```python
from build123d import *

# Parameters (mm, degrees)
SKETCH1_W                = 12.5984
SKETCH1_H                = 13.4112
BOSS_EXTRUDE1_DEPTH      = 46.99
BOSS_EXTRUDE1_DEPTH_BACK = 39.37
SKETCH2_R                = 3.1242
CUT_EXTRUDE1_DEPTH       = 87.36
SKETCH4_R                = 2.54
BOSS_EXTRUDE2_DEPTH      = 2.54
FILLET2_R                = 0.508
FILLET2_OF_MIRROR1_R     = 0.508
FILLET1_R                = 1.778
CHAMFER1_SIZE            = 1.27


with BuildPart() as part:
    # Sketch1 → Boss-Extrude1 (new body, two sides)
    with BuildSketch(Plane(origin=(0, 0, 0), x_dir=(1, 0, 0), z_dir=(0, 1, 0))) as boss_extrude1_sk:
        with Locations((-1.1938, -0.7874)):
            Rectangle(SKETCH1_W, SKETCH1_H)
    extrude(amount=BOSS_EXTRUDE1_DEPTH)
    extrude(boss_extrude1_sk.sketch, amount=-BOSS_EXTRUDE1_DEPTH_BACK)

    # Sketch2 → Cut-Extrude1 (cut, through all)
    with BuildSketch(Plane(origin=(0, 46.99, 0), x_dir=(1, 0, 0), z_dir=(0, 1, 0))):
        with Locations(Location((0, 0, 0), (0, 0, 270))):  # turned: the seam where the file's is
            Circle(SKETCH2_R)
    extrude(amount=-CUT_EXTRUDE1_DEPTH, mode=Mode.SUBTRACT)

    # Sketch4 → Boss-Extrude2 (add)
    with BuildSketch(Plane(origin=(5.1054, 0, 0), x_dir=(0, 0, -1), z_dir=(1, 0, 0))):
        with Locations((0, -20.32)):
            Circle(SKETCH4_R)
    boss_extrude2 = extrude(amount=BOSS_EXTRUDE2_DEPTH)

    # Fillet2
    fillet2_edges = [part.edges().sort_by_distance(p)[0] for p in [
        (7.6454, -20.32, 2.54),
    ]]
    fillet(fillet2_edges, radius=FILLET2_R)

    # Mirror1: Boss-Extrude2 across plane
    add(boss_extrude2.mirror(Plane.ZX))

    # Fillet2 of Mirror1
    fillet2_of_mirror1_edges = [part.edges().sort_by_distance(p)[0] for p in [
        (7.6454, 20.32, 2.54),
    ]]
    fillet(fillet2_of_mirror1_edges, radius=FILLET2_OF_MIRROR1_R)

    # Fillet1
    fillet1_edges = [part.edges().sort_by_distance(p)[0] for p in [
        (5.1054, 3.81, -5.9182),
        (-7.493, 3.81, 7.493),
    ]]
    fillet(fillet1_edges, radius=FILLET1_R)

    # Chamfer1
    chamfer1_edges = [part.edges().sort_by_distance(p)[0] for p in [
        (0, 46.99, -3.1242),
    ]]
    chamfer(chamfer1_edges, length=CHAMFER1_SIZE)


solid = part.part
```
For this review, take the finished solid that the model builds, in its own axes (mm). A direction names the side the tool comes from. Round coordinates to 2 decimals unless told otherwise and drop trailing zeros. Loops run counter-clockwise (first coordinate to the right, second up) from the corner with the lowest first, then second, coordinate; pieces in that order, holes last.
Q1. To check wall thickness, follow line 1 along X through (y, z) = (17, 0); line 2 along X through (y, z) = (-35.5, -2.5); line 3 along Z through (x, y) = (2, -4). State the ranges of each line that lie inside material, in increasing order.
Result sheet:
line 1: x = -7.49 to -3.12, 3.12 to 5.11
line 2: x = -7.49 to -1.87, 1.87 to 5.11
line 3: z = -5.92 to -2.4, 2.4 to 7.49
Q2. Add section A-A on y = -20.32. Write out the cut boundary in (x, z) (3 decimals), plus the area to 3 significant figures.
Result sheet:
outline: (-7.493, -5.918) - (3.327, -5.918) arc R1.778 ccw to (5.105, -4.14) - (5.105, -2.54) - (7.137, -2.54) arc R0.508 ccw to (7.645, -2.032) - (7.645, 2.032) arc R0.508 ccw to (7.137, 2.54) - (5.105, 2.54) - (5.105, 7.493) - (-5.715, 7.493) arc R1.778 ccw to (-7.493, 5.715) - close; hole circle Ø6.248 at (0, 0)
area: 150 mm2
Q3. Add section B-B on x = 0. Write out the cut boundary in (y, z), plus the area to 3 significant figures.
Result sheet:
outline: (-39.37, -5.92) - (46.99, -5.92) - (46.99, -4.39) - (45.72, -3.12) - (-39.37, -3.12) - close; (-39.37, 3.12) - (45.72, 3.12) - (46.99, 4.39) - (46.99, 7.49) - (-39.37, 7.49) - close
area: 617 mm2
Q4. Add section D-D on y = 37.5. Write out the cut boundary in (x, z) (3 decimals).
Result sheet:
outline: (-7.493, -5.918) - (3.327, -5.918) arc R1.778 ccw to (5.105, -4.14) - (5.105, 7.493) - (-5.715, 7.493) arc R1.778 ccw to (-7.493, 5.715) - close; hole circle Ø6.248 at (0, 0)
Q5. Mouldability with a two-part tool opening along Y and no side actions: class faces 3 (the face through (0.94, 3.77, 2.98)), 4 (the face through (6.11, 17.8, 0.33)), 5 (the face through (-3, -39.37, 2)) as +Y half, -Y half, draft (parallel to the pull), parting line (faces both ways), or undercut.
Result sheet:
face 3: draft
face 4: undercut
face 5: -Y half
Q6. Machinability: for faces 1 (the face through (4.6, 3.21, -5.38)), 2 (the face through (6.11, -17.8, 0.33)), which of the approach directions +Z, -Z, +X, -X, +Y, -Y give a long, thin tool a straight path to every point of the face, cutting with its end or side? Answer none if there is none.
Result sheet:
face 1: -Z, +X, +Y, -Y
face 2: +X
Q7. Insertion check: pin 1 Ø6 at (x, z) = (-0.5, -3) entering from +Y; pin 2 Ø5 at (x, z) = (0, 0) entering from -Y. Each pin has a flat end and moves straight along its axis. Give the tip position at first contact, or say it passes through.
Result sheet:
pin 1: stops at y = 46.99
pin 2: passes through
Q8. Add section C-C on z = 0. Write out the cut boundary in (x, y).
Result sheet:
outline: (-7.49, -39.37) - (-3.12, -39.37) - (-3.12, 45.72) - (-4.39, 46.99) - (-7.49, 46.99) - close; (3.12, -39.37) - (5.11, -39.37) - (5.11, -22.86) - (7.14, -22.86) arc R0.51 ccw to (7.65, -22.35) - (7.65, -18.29) arc R0.51 ccw to (7.14, -17.78) - (5.11, -17.78) - (5.11, 17.78) - (7.14, 17.78) arc R0.51 ccw to (7.65, 18.29) - (7.65, 22.35) arc R0.51 ccw to (7.14, 22.86) - (5.11, 22.86) - (5.11, 46.99) - (4.39, 46.99) - (3.12, 45.72) - close
